Source: CAD feature listing. Evaluate the final solid. Frame: model axes, mm. A direction names the side the tool comes from. Coordinates: 2 decimals unless noted, no trailing zeros. Write each loop counter-clockwise with the first axis right and the second up, starting at its lowest first coordinate (ties: lowest second). Pieces come first, ordered by that corner, then holes. Notation, with made-up numbers: (75, 44) - (103, 44) arc R22 cw to (103, 71) - close; hole circle Ø7 at (63.25, 65.5). An arc over 180 degrees is marked (long way). One line per item, written item: value.
Autodesk Inventor part; units mm, degrees
ref_plane "Work Plane1" through (0, 25, 0) normal (0, 1, 0) x (-1, 0, 0)
ref_plane "YZ Plane" through (0, 0, 0) normal (1, 0, 0) x (0, 1, 0)
ref_plane "XY Plane" through (0, 0, 0) normal (0, 0, 1) x (1, 0, 0)
sketch "Sketch1" plane through (0, 0, 0) normal (0, 0, 1) x (1, 0, 0)
  arc A0 (14.865, 0) -> (-14.865, 0) centre (0, 0) ccw
  arc A1 (17.1039, 3) -> (-17.1039, 3) centre (0, 0) ccw
  line L0 (-17.1039, 3) -> (-29.865, 3)
  line L1 (-29.865, 3) -> (-29.865, 0)
  line L2 (-29.865, 0) -> (-14.865, 0)
  line L3 (14.865, 0) -> (29.865, 0)
  line L4 (29.865, 0) -> (29.865, 3)
  line L5 (29.865, 3) -> (17.1039, 3)
  dimension "d0" = 3
  dimension "d1" = 14.865
  dimension "d2" = 2.5
  dimension "d3" = 15
extrude "Extrusion1" add sketch "Sketch1" along normal blind 15
sketch "Sketch2" plane through (-29.865, 0, 0) normal (0, -1, 0) x (1, 0, 0)
  line L0 (0, 15) -> (15, 15)
  line L1 (0, 0) -> (0, 15)
  point P0 (29.865, 0)
  point P1 (7.5, 7.5)
  point P2 (7.5, 15)
  point P3 (0, 7.5)
hole "Hole1" at (-22.365, 0, 7.5) direction (0, 1, 0) diameter 3 end through all
mirror "Mirror1" about plane through (0, 0, 0) normal (1, 0, 0) of "Hole1"
ref_plane "Work Plane1" through (0, 25, 0) normal (0, 1, 0) x (-1, 0, 0)
sketch "Sketch3" plane through (0, 25, 0) normal (0, 1, 0) x (-1, 0, 0)
  line L0 (-17.1039, 0) -> (17.1039, 0)
  line L1 (-17.1039, 0) -> (-17.1039, 15)
  line L2 (17.1039, 0) -> (17.1039, 15)
  line L3 (-17.1039, 15) -> (-14.1039, 15)
  line L4 (17.1039, 15) -> (14.1039, 15)
  arc A0 (-14.1039, 15) -> (14.1039, 15) centre (0, 17.2883) ccw
  point P0 (0, 0)
  point P1 (0, 3)
  dimension "d14" = 3
  dimension "d15" = 3
  dimension "d16" = 3
extrude "Extrusion2" add sketch "Sketch3" against normal up to next
fillet "Fillet1" radius 4 4 edges at (-29.865, 1.5, 15) (-29.865, 1.5, 0) (29.865, 1.5, 0) (29.865, 1.5, 15)
properties part number "Motor Mount C-Clamp Base"
1) Material intervals for line 1 (X direction, y = 0.95, z = 7.5) (3 decimals); line 2 (X direction, y = 15.75, z = 7.75); line 3 (X direction, y = 13.5, z = 12.5), sorted ascending.
Values found:
line 1: -29.865 to -23.865, -20.865 to -14.835, 14.835 to 20.865, 23.865 to 29.865
line 2: -17.1 to -10.64, -7.31 to 7.31, 10.64 to 17.1
line 3: -17.1 to -13.46, -10.92 to -6.22, 6.22 to 10.92, 13.46 to 17.1
2) Section query D-D on y = 16.5. Output: boundary loops of the cut face in (x, z).
Values found:
outline: (-17.1, 0) - (17.1, 0) - (17.1, 15) - (14.1, 15) arc R14.29 cw to (5.41, 4.06) - (5.41, 15) - (-5.41, 15) - (-5.41, 4.06) arc R14.29 cw to (-14.1, 15) - (-17.1, 15) - close
3) Contact query for flat-ended pins moving along their axis: P1, Ø4, axis at x = 2.5, y = 19.5, coming from the -Z side; P2, Ø2, axis at x = -9.5, z = 13, coming from the -Y side; P3, Ø2.5, axis at x = 22.365, z = 7.5, coming from the -Y side; P4, Ø2, axis at y = 9, z = 11.5, coming from the -X side. Output: stop coordinate, or through.
Values found:
P1: z = 0
P2: y = 10.52
P3: through
P4: x = -17.1
4) Section query A-A on y = 7.5. Output: boundary loops of the cut face in (x, z).
Values found:
outline: (-17.1, 0) - (-12.83, 0) - (-12.83, 15) - (-17.1, 15) - close; (12.83, 0) - (17.1, 0) - (17.1, 15) - (12.83, 15) - close
5) Section query B-B on z = 7.5. Output: boundary loops of the cut face in (x, y) (3 decimals), then the cut area to 3 significant figures.
Values found:
outline: (-29.865, 0) - (-23.865, 0) - (-23.865, 3) - (-29.865, 3) - close; (-20.865, 0) - (-14.865, 0) arc R14.865 cw to (14.865, 0) - (20.865, 0) - (20.865, 3) - (17.104, 3) - (17.104, 25) - (10.409, 25) - (10.409, 13.9) arc R17.365 ccw to (-10.409, 13.9) - (-10.409, 25) - (-17.104, 25) - (-17.104, 3) - (-20.865, 3) - close; (23.865, 0) - (29.865, 0) - (29.865, 3) - (23.865, 3) - close
area: 385 mm2
6) Reachability of faces 4 (the flat face through (-17.104, 14, 7)), 5 (the cylindrical face through (-21.45, 1.52, 8.69)), 6 (the flat face through (25, 3, 7)) from +Z, -Z, +X, -X, +Y, -Y: full face, straight path, thin tool, end or side. Return the list, or none.
Values found:
face 4: +Z, -Z, -X, +Y
face 5: +Y, -Y
face 6: +Z, -Z, +X, +Y
7) Draft query along X for faces 1 (the cylindrical face through (-0.33, 14.86, 7.4)), 2 (the flat face through (5, 15, 0)), 3 (the flat face through (17.104, 14, 7)). Return one class per face: released by +X, released by -X, zero draft, split by the parting line, or undercut.
Values found:
face 1: undercut
face 2: zero draft
face 3: released by +X
8) Section query C-C on x = 0. Output: boundary loops of the cut face in (y, z) (3 decimals).
Values found:
outline: (14.865, 0) - (25, 0) - (25, 3) - (17.365, 3) - (17.365, 15) - (14.865, 15) - close
